from build123d import *

# Parameters (mm, degrees)
SKETCH1_R           = 2.5
BOSS_EXTRUDE1_DEPTH = 33
FILLET1_R           = 1


with BuildPart() as part:
    # Sketch1 → Boss-Extrude1 (new body)
    with BuildSketch(Plane(origin=(0, 0, 0), x_dir=(0, 0, -1), z_dir=(1, 0, 0))):
        with BuildLine():
            Line((-16, 22), (16, 22))
            ThreePointArc((16, 22), (20.242640687, 20.242640687), (22, 16))
            Line((22, 16), (22, -16))
            ThreePointArc((22, -16), (20.242640687, -20.242640687), (16, -22))
            Line((16, -22), (-16, -22))
            ThreePointArc((-16, -22), (-20.242640687, -20.242640687), (-22, -16))
            Line((-22, -16), (-22, 16))
            ThreePointArc((-22, 16), (-20.242640687, 20.242640687), (-16, 22))
        make_face()
        Circle(SKETCH1_R, mode=Mode.SUBTRACT)
    extrude(amount=BOSS_EXTRUDE1_DEPTH)

    # Fillet1
    fillet1_edges = [part.edges().sort_by_distance(p)[0] for p in [
        (0, 0, -22),
        (0, -20.242640687, -20.242640687),
        (0, -22, 0),
        (0, -20.242640687, 20.242640687),
        (33, -20.242640687, -20.242640687),
        (33, 0, -22),
        (33, 20.242640687, -20.242640687),
        (33, 22, 0),
        (33, 20.242640687, 20.242640687),
        (33, 0, 22),
        (33, -20.242640687, 20.242640687),
        (0, 0, 22),
        (33, -22, 0),
        (0, 20.242640687, 20.242640687),
        (0, 22, 0),
        (0, 20.242640687, -20.242640687),
    ]]
    fillet(fillet1_edges, radius=FILLET1_R)


solid = part.part
Check sheet for the modelled part. Datum: model origin and axes. Units: mm. Give positions to 0.01 mm unless a question says otherwise; leave off trailing zeros. Loops run counter-clockwise (first coordinate to the right, second up) from the corner with the lowest first, then second, coordinate; pieces in that order, holes last. Notation, with made-up numbers: M 67,78.5 L 99,78.5 A22 ccw 99,84.5 Z; hole C 44,-17 d9. An arc over 180 degrees is marked long. Answer as a JSON object with one key per item and string values. Group by question number.
Q1. Cross-section at A-A on z = 0. Record the cut outline in (x, y).
Q2. Cross-section at C-C on x = 18. Record the cut outline in (y, z).
Q3. Release check for a two-part mould opening along Z. For faces 1 (the cylindrical face through (16.283, -20.196, -20.289)), 2 (the flat face through (16, -22, 0)), 3 (the cylindrical face through (16.27, -2.44, 0.54)), 4 (the cylindrical face through (16.283, -20.289, 20.196)) record: released by +Z, released by -Z, zero draft, split by the parting line, or undercut.
Q4. Material ranges on line 1 along Y through (x, z) = (12, 0); line 2 along Y through (x, z) = (27, 0.5); line 3 along Y through (x, z) = (14.5, -18.5), recorded low to high. Write a range as [from, to].
Evaluation:
{
 "1": {"outline": "M 0,-21 A1 ccw 1,-22 L 32,-22 A1 ccw 33,-21 L 33,-2.5 L 0,-2.5 Z; M 0,2.5 L 33,2.5 L 33,21 A1 ccw 32,22 L 1,22 A1 ccw 0,21 Z"},
 "2": {"outline": "M -22,-16 A6 ccw -16,-22 L 16,-22 A6 ccw 22,-16 L 22,16 A6 ccw 16,22 L -16,22 A6 ccw -22,16 Z; hole C 0,0 d5"},
 "3": {"face 1": "released by -Z", "face 2": "zero draft", "face 3": "undercut", "face 4": "released by +Z"},
 "4": {"line 1": "y = [-22, -2.5], [2.5, 22]", "line 2": "y = [-22, -2.45], [2.45, 22]", "line 3": "y = [-21.45, 21.45]"}
}
